CAD build for the part. Positions are in the model's coordinates, mm. Face numbers are marked on the shaded views. A direction names the side the tool comes from. Coordinates: 2 decimals unless noted, no trailing zeros. Order: outer loops, then holes, each group sorted by start corner. A loop starts at its lowest first (then second) coordinate and runs counter-clockwise, first axis right, second up. Notation, with made-up numbers: (-6, 0.25) - (48, 0.25) arc R19 cw to (48, 16.25) - close; hole circle Ø4 at (8, 35). An arc over 180 degrees is marked (long way). Write each question's results on one line, items separated by ' | '. Start each with the question number.
Q1. Band-saw the part on A-A, the plane y = 32.5. Write the cut outline in (x, z).
Q2. Pin check, flat tips, straight feed: P1, Ø5, axis at y = 18, z = 6.5, coming from the -X side; P2, Ø1.7, axis at x = -13, z = 6.5, coming from the +Y side; P3, Ø1, axis at x = 15, y = 22.5, coming from the +Z side; P4, Ø24, axis at x = 1.5, z = -3.5, coming from the -Y side. Stop position of each tip, or through.
Q3. Pull direction Z, two halves, no side cores. Call the marked faces 6, 7 and 8: released by +Z, released by -Z, zero draft, split by the parting line, or undercut.
Q4. Wall check: probe 1 along X at (y, z) = (46.1, 0); probe 2 along Z at (x, y) = (0, 5.5); probe 3 along Z at (x, y) = (0, 1.3). Give the ranges that are in metal, low to high.
Q5. Which spindle directions (+Z, -Z, +X, -X, +Y, -Y) get a long thin tool onto all of the face, cutting with end or side? Do the marked faces 1, 2, 3, 4 and 5. Say none if no direction does.
Q6. Band-saw the part on B-B, the plane y = 20.5. Write the cut outline in (x, z), then the cut area to 3 significant figures.
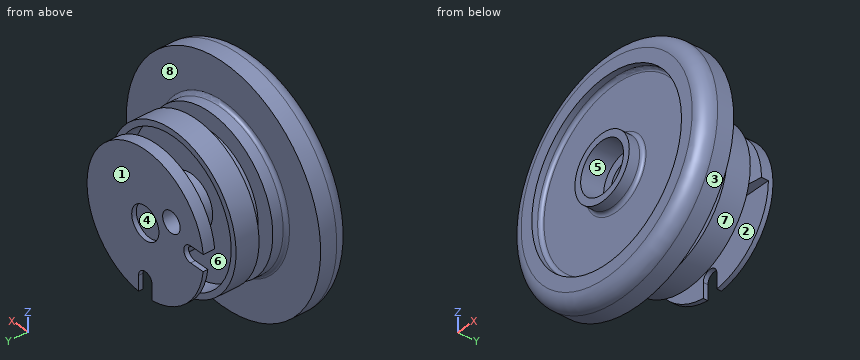
```python
from build123d import *

# Parameters (mm, degrees)
CROQUIS1_R               = 50
SALIENTE_EXTRUIR1_DEPTH  = 13
CROQUIS1_3_R             = 38.5
CORTAR_EXTRUIR1_DEPTH    = 4
CROQUIS4_R               = 14
CROQUIS4_R_2             = 11
SALIENTE_EXTRUIR3_DEPTH  = 6
CROQUIS4_2_R             = 11
CORTAR_EXTRUIR4_DEPTH    = 10
REDONDEO1_R              = 1.5
REDONDEO2_R              = 1.5
REDONDEO3_R              = 6
CROQUIS7_R               = 32.5
CROQUIS7_R_2             = 11
SALIENTE_EXTRUIR4_DEPTH  = 6
REDONDEO4_R              = 1.5
CROQUIS9_R               = 25
CROQUIS9_R_2             = 11
SALIENTE_EXTRUIR6_DEPTH  = 6
CROQUIS10_R              = 32.5
CROQUIS10_R_2            = 11
SALIENTE_EXTRUIR7_DEPTH  = 10
CROQUIS11_R              = 30
CROQUIS11_R_2            = 11
CORTAR_EXTRUIR5_DEPTH    = 8
CROQUIS12_R              = 11
CROQUIS12_R_2            = 7
SALIENTE_EXTRUIR8_DEPTH  = 29
CROQUIS12_2_R            = 11
CROQUIS12_2_R_2          = 7
SALIENTE_EXTRUIR9_DEPTH  = 18
CROQUIS13_R              = 11
CORTAR_EXTRUIR6_DEPTH    = 10
CROQUIS14_R              = 15
SALIENTE_EXTRUIR11_DEPTH = 10
SALIENTE_EXTRUIR12_DEPTH = 8
CORTAR_REVOLUCI_N1_ANGLE = 180
CROQUIS19_R              = 30
CROQUIS19_R_2            = 7
SALIENTE_EXTRUIR13_DEPTH = 2
CORTAR_EXTRUIR9_DEPTH    = 10
CROQUIS21_R              = 4.5
CORTAR_EXTRUIR10_DEPTH   = 10


with BuildPart() as part:
    # Croquis1 → Saliente-Extruir1 (new body)
    with BuildSketch(Plane(origin=(0, 0, 0), x_dir=(1, 0, 0), z_dir=(0, 1, 0))):
        Circle(CROQUIS1_R)
    extrude(amount=SALIENTE_EXTRUIR1_DEPTH)

    # Croquis1<3> → Cortar-Extruir1 (cut)
    with BuildSketch(Plane(origin=(0, 0, 0), x_dir=(1, 0, 0), z_dir=(0, 1, 0))):
        Circle(CROQUIS1_3_R)
    extrude(amount=CORTAR_EXTRUIR1_DEPTH, mode=Mode.SUBTRACT)

    # Croquis4 → Saliente-Extruir3 (add)
    with BuildSketch(Plane.XZ.offset(-4)):
        Circle(CROQUIS4_R)
        Circle(CROQUIS4_R_2, mode=Mode.SUBTRACT)
    extrude(amount=SALIENTE_EXTRUIR3_DEPTH)

    # Croquis4<2> → Cortar-Extruir4 (cut, through all)
    with BuildSketch(Plane.XZ.offset(-4)):
        Circle(CROQUIS4_2_R)
    extrude(amount=-CORTAR_EXTRUIR4_DEPTH, mode=Mode.SUBTRACT)

    # Redondeo1
    redondeo1_edges = [part.edges().sort_by_distance(p)[0] for p in [
        (-38.5, 4, 0),
    ]]
    fillet(redondeo1_edges, radius=REDONDEO1_R)

    # Redondeo2
    redondeo2_edges = [part.edges().sort_by_distance(p)[0] for p in [
        (-14, 4, 0),
    ]]
    fillet(redondeo2_edges, radius=REDONDEO2_R)

    # Redondeo3
    redondeo3_edges = [part.edges().sort_by_distance(p)[0] for p in [
        (-50, 0, 0),
    ]]
    fillet(redondeo3_edges, radius=REDONDEO3_R)

    # Croquis7 → Saliente-Extruir4 (add)
    with BuildSketch(Plane(origin=(0, 13, 0), x_dir=(1, 0, 0), z_dir=(0, 1, 0))):
        Circle(CROQUIS7_R)
        Circle(CROQUIS7_R_2, mode=Mode.SUBTRACT)
    extrude(amount=SALIENTE_EXTRUIR4_DEPTH)

    # Redondeo4
    redondeo4_edges = [part.edges().sort_by_distance(p)[0] for p in [
        (-32.5, 13, 0),
    ]]
    fillet(redondeo4_edges, radius=REDONDEO4_R)

    # Croquis9 → Saliente-Extruir6 (add)
    with BuildSketch(Plane(origin=(0, 19, 0), x_dir=(1, 0, 0), z_dir=(0, 1, 0))):
        Circle(CROQUIS9_R)
        Circle(CROQUIS9_R_2, mode=Mode.SUBTRACT)
    extrude(amount=SALIENTE_EXTRUIR6_DEPTH)

    # Croquis10 → Saliente-Extruir7 (add)
    with BuildSketch(Plane(origin=(0, 25, 0), x_dir=(1, 0, 0), z_dir=(0, 1, 0))):
        Circle(CROQUIS10_R)
        Circle(CROQUIS10_R_2, mode=Mode.SUBTRACT)
    extrude(amount=SALIENTE_EXTRUIR7_DEPTH)

    # Croquis11 → Cortar-Extruir5 (cut)
    with BuildSketch(Plane(origin=(0, 35, 0), x_dir=(1, 0, 0), z_dir=(0, 1, 0))):
        Circle(CROQUIS11_R)
        Circle(CROQUIS11_R_2, mode=Mode.SUBTRACT)
    extrude(amount=-CORTAR_EXTRUIR5_DEPTH, mode=Mode.SUBTRACT)

    # Croquis12 → Saliente-Extruir8 (add, through all)
    with BuildSketch(Plane(origin=(0, 27, 0), x_dir=(1, 0, 0), z_dir=(0, 1, 0))):
        Circle(CROQUIS12_R)
        Circle(CROQUIS12_R_2, mode=Mode.SUBTRACT)
    extrude(amount=-SALIENTE_EXTRUIR8_DEPTH)

    # Croquis12<2> → Saliente-Extruir9 (add)
    with BuildSketch(Plane(origin=(0, 27, 0), x_dir=(1, 0, 0), z_dir=(0, 1, 0))):
        Circle(CROQUIS12_2_R)
        Circle(CROQUIS12_2_R_2, mode=Mode.SUBTRACT)
    extrude(amount=SALIENTE_EXTRUIR9_DEPTH)

    # Croquis13 → Cortar-Extruir6 (cut)
    with BuildSketch(Plane.XZ.offset(2)):
        Circle(CROQUIS13_R)
    extrude(amount=-CORTAR_EXTRUIR6_DEPTH, mode=Mode.SUBTRACT)

    # Croquis14 → Saliente-Extruir11 (add)
    with BuildSketch(Plane(origin=(0, 45, 0), x_dir=(1, 0, 0), z_dir=(0, 1, 0))):
        Circle(CROQUIS14_R)
    extrude(amount=-SALIENTE_EXTRUIR11_DEPTH)

    # Croquis17 → Saliente-Extruir12 (add)
    with BuildSketch(Plane(origin=(0, 45, 0), x_dir=(1, 0, 0), z_dir=(0, 1, 0))):
        with BuildLine():
            Line((30, 0), (15, 0))
            ThreePointArc((15, 0), (0, -15), (-15, 0))
            Line((-15, 0), (-30, 0))
            ThreePointArc((-30, 0), (0, -30), (30, 0))
        make_face()
    extrude(amount=-SALIENTE_EXTRUIR12_DEPTH)

    # Croquis18 → Cortar-Revolución1 (revolve, cut)
    with BuildSketch(Plane(origin=(0, 0, 0), x_dir=(-1, 0, 0), z_dir=(0, 0, -1))):
        Polygon((15, 40), (30, 42), (30, 37), (15, 37), align=None)
    revolve(axis=Axis((0, 37, 0), (0, 1, 0)), revolution_arc=CORTAR_REVOLUCI_N1_ANGLE, mode=Mode.SUBTRACT)

    # Croquis19 → Saliente-Extruir13 (add)
    with BuildSketch(Plane(origin=(0, 45, 0), x_dir=(1, 0, 0), z_dir=(0, 1, 0))):
        Circle(CROQUIS19_R)
        Circle(CROQUIS19_R_2, mode=Mode.SUBTRACT)
    extrude(amount=SALIENTE_EXTRUIR13_DEPTH)

    # Croquis20 → Cortar-Extruir9 (cut)
    with BuildSketch(Plane(origin=(0, 47, 0), x_dir=(1, 0, 0), z_dir=(0, 1, 0))):
        with BuildLine():
            Line((3.505959936, 29.79443312), (3.505959936, 23.29443312))
            ThreePointArc((3.505959936, 23.29443312), (0.005959936, 19.79443312), (-3.494040064, 23.29443312))
            Line((-3.494040064, 23.29443312), (-3.494040064, 29.795833333))
            ThreePointArc((-3.494040064, 29.795833333), (0.006000915, 29.9999994), (3.505959936, 29.79443312))
        make_face()
        with BuildLine():
            Line((-29.79443312, 3.505959936), (-23.29443312, 3.505959936))
            ThreePointArc((-23.29443312, 3.505959936), (-19.79443312, 0.005959936), (-23.29443312, -3.494040064))
            Line((-23.29443312, -3.494040064), (-29.795833333, -3.494040064))
            ThreePointArc((-29.795833333, -3.494040064), (-29.9999994, 0.006000915), (-29.79443312, 3.505959936))
        make_face()
    extrude(amount=-CORTAR_EXTRUIR9_DEPTH, mode=Mode.SUBTRACT)

    # Croquis21 → Cortar-Extruir10 (cut)
    with BuildSketch(Plane(origin=(0, 47, 0), x_dir=(1, 0, 0), z_dir=(0, 1, 0))):
        with Locations((-13.423393759, -7.75)):
            Circle(CROQUIS21_R)
    extrude(amount=-CORTAR_EXTRUIR10_DEPTH, mode=Mode.SUBTRACT)


solid = part.part
```
Results below:
1) outline: circle Ø65 at (0, 0); circle Ø22 at (0, 0); hole circle Ø60 at (0, 0); hole circle Ø14 at (0, 0)
2) P1: stops at x = -32.25 | P2: stops at y = 37 | P3: stops at z = 20.37 | P4: stops at y = -2
3) face 6: undercut | face 7: split by the parting line | face 8: zero draft
4) probe 1: x = -19.79 to -7, 7 to 30 | probe 2: z = -49.98 to -11, 11 to 49.98 | probe 3: z = -47.73 to -38.5, -14 to -11, 11 to 14, 38.5 to 47.73
5) face 1: +Z, -Z, +X, -X, +Y | face 2: -Z | face 3: +Y, -Y | face 4: +Y | face 5: -Y
6) outline: circle Ø50 at (0, 0); hole circle Ø14 at (0, 0) | area: 1,810 mm²
